```python
from build123d import *

# Parameters (mm, degrees)
F1_DEPTH  = 32
F3_DEPTH  = 1.5
F2_W      = 6
F2_H      = 19
F4_DEPTH  = 2
F5_W      = 60
F5_H      = 27.5
F6_DEPTH  = 1.5
F7_SIZE   = 1.49999
F8_SIZE   = 0.5
F10_DEPTH = 2


# Not quite as in the source:
# - a fillet or chamfer is up to 0.001 mm smaller than in the source, because OpenCascade refuses the exact size


with BuildPart() as f1:
    # F0 (on Right) → F1 (new body, symmetric)
    with BuildSketch(Plane.YZ):
        Polygon((-12.5, 0), (-12.5, 29.5), (12.5, 29.5), (12.5, 3), (14.5, 3), (14.5, 31.5), (-14.5, 31.5), (-14.5, 0), align=None)
    extrude(amount=F1_DEPTH, both=True)

    # F2 (on face) → F3 (cut)
    with BuildSketch(Plane(origin=(0, 14.5, 0), x_dir=(-1, 0, 0), z_dir=(0, 1, 0))):
        Polygon((-9, 5), (30, 5), (30, 29.5), (-30, 29.5), (-30, 5), (-19, 5), (-19, 24), (-9, 24), align=None)
    extrude(amount=-F3_DEPTH, mode=Mode.SUBTRACT)

    # F2 (on face) → F4 (cut)
    with BuildSketch(Plane(origin=(0, 14.5, 0), x_dir=(-1, 0, 0), z_dir=(0, 1, 0))):
        with Locations((-14, 12.5)):
            Rectangle(F2_W, F2_H)
    extrude(amount=-F4_DEPTH, mode=Mode.SUBTRACT)

    # F5 (on face) → F6 (cut)
    with BuildSketch(Plane.XZ.offset(14.5)):
        with Locations((0, 15.75)):
            Rectangle(F5_W, F5_H)
    extrude(amount=-F6_DEPTH, mode=Mode.SUBTRACT)

    # F7 (size 1.5 in the source; OpenCascade refuses exactly that, so slightly less here)
    f7_edges = [f1.edges().sort_by_distance(p)[0] for p in [
        (-30, 13, 17.25),
        (0, 13, 29.5),
        (30, 13, 17.25),
        (9, 13, 14.5),
        (-10.5, 13, 5),
        (24.5, 13, 5),
        (19, 13, 14.5),
        (14, 13, 24),
        (0, -13, 29.5),
        (-30, -13, 15.75),
        (0, -13, 2),
        (30, -13, 15.75),
    ]]
    chamfer(f7_edges, length=F7_SIZE)

    # F8
    f8_edges = [f1.edges().sort_by_distance(p)[0] for p in [
        (0, 14.5, 31.5),
        (0, -14.5, 31.5),
        (32, 0, 31.5),
        (-32, 0, 31.5),
    ]]
    chamfer(f8_edges, length=F8_SIZE)

    # F9 (on face) → F10 (cut)
    with BuildSketch(Plane.XY.offset(31.5)):
        Polygon((27.9455012138, 11.5), (-27.9455012138, 11.5), (0, 1.0674114154), align=None)
        Polygon((-2.8592469416, 0), (-29.5, 9.9455012138), (-29.5, -9.9455012138), align=None)
        Polygon((0, -1.0674114154), (-27.9455012138, -11.5), (27.9455012138, -11.5), align=None)
        Polygon((29.5, -9.9455012138), (29.5, 9.9455012138), (2.8592469416, 0), align=None)
    extrude(amount=-F10_DEPTH, mode=Mode.SUBTRACT)


solid = f1.part
```
Geometry check sheet. Reference: the model listing, model coordinates, mm. A direction names the side the tool comes from. Give positions to 0.01 mm unless a question says otherwise; leave off trailing zeros. Order: outer loops, then holes, each group sorted by start corner. A loop starts at its lowest first (then second) coordinate and runs counter-clockwise, first axis right, second up.
1. Section check B-B, the plane y = 8.75. Enter the section's corners in (x, z).
2. Release check for a two-part mould opening along Z. For faces 6 (the face through (-10, 13, 3)), 7 (the face through (32, -1, 30)), 8 (the face through (-29.2, -13.7, 15.6)) record: pulls with the +Z half, pulls with the -Z half, needs draft (parallel to the pull), parting line crosses it, or undercut.
3. Access from +Z, -Z, +X, -X, +Y, -Y to the whole of each face (thin tool, end or side, straight path). Record for faces 1 (the face through (0, -13, 16)), 2 (the face through (-16.366, -5.042, 30.514)), 3 (the face through (0, 12.5, 16)), 4 (the face through (-6, 13, 17)), 5 (the face through (17, 14, 12)).
4. Thickness scan on L1, parallel to Y at x = -6, z = 23; L2, parallel to Y at x = 29.5, z = 25; L3, parallel to Z at x = -3, y = -12. Record the ranges inside material, lowest first.
5. Gauge pin test, flat ends, axial feed: pin 1 Ø1.6 at (x, y) = (26.5, 13) entering from -Z; pin 2 Ø2 at (x, y) = (12.5, 13.5) entering from -Z; pin 3 Ø12 at (x, y) = (17, 5) entering from -Z. Record the tip position at first contact, or that the pin passes through.
6. Section check A-A, the plane z = 17. Give the number of separate pieces and of enclosed holes in the cut face, and give its area (4 significant figures).
Values follow:
1. outline: (-32, 29.5) - (-29.5, 29.5) - (-29.5, 31.5) - (-31.5, 31.5) - (-32, 31) - close; (-26.3, 29.5) - (-20.58, 29.5) - (-20.58, 31.5) - (-26.3, 31.5) - close; (20.58, 29.5) - (26.3, 29.5) - (26.3, 31.5) - (20.58, 31.5) - close; (29.5, 29.5) - (32, 29.5) - (32, 31) - (31.5, 31.5) - (29.5, 31.5) - close
2. face 6: pulls with the -Z half
2. face 7: needs draft
2. face 8: undercut
3. face 1: -Y
3. face 2: +Z, -Z
3. face 3: -Z, +X, -X
3. face 4: +Y
3. face 5: -Z, +Y
4. L1: y = -13 to -12.5, 12.5 to 13
4. L2: y = -14 to -12.5, 12.5 to 14
4. L3: z = 29.5 to 31.5
5. pin 1: stops at z = 3
5. pin 2: stops at z = 22
5. pin 3: stops at z = 29.5
6. separate pieces: 3
6. enclosed holes: 0
6. area: 85.75 mm2
